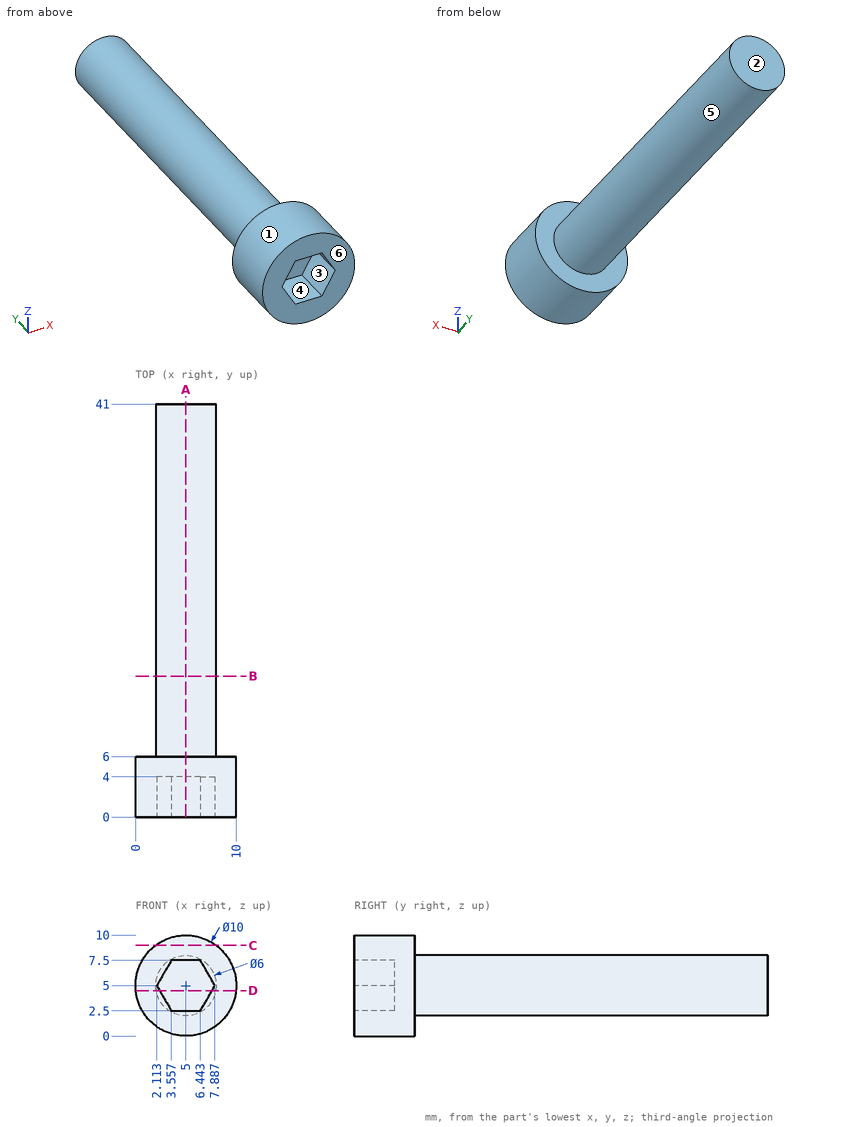
Geometry: see drawing. Coordinates: mm, zero at the bounding-box minimum. A direction names the side the tool comes from. Round coordinates to 2 decimals unless told otherwise and drop trailing zeros. Loops run counter-clockwise (first coordinate to the right, second up) from the corner with the lowest first, then second, coordinate; pieces in that order, holes last. Notation, with made-up numbers: (82, 79) - (130, 79) arc R27 cw to (130, 100) - close; hole circle Ø9 at (2.5, 38). An arc over 180 degrees is marked (long way). Write item = value, one per line. Start each with the question number.
(1) Set-up query: the marked faces 4, 5 and 6. Return all of +Z, -Z, +X, -X, +Y, -Y with unobstructed straight access to the full face (end or side cutting, diameter ignored); none if empty.
(2) Section query C-C, the plane z = 9. Output: boundary loops of the cut face in (x, y).
(3) Section query A-A, the plane x = 5. Output: boundary loops of the cut face in (y, z), plus the area to 3 significant figures.
(4) Section query B-B, the plane y = 14. Output: boundary loops of the cut face in (x, z).
(5) Pull-direction query (X, two-part tool) for the marked faces 1, 2 and 3; classes: +X half, -X half, draft (parallel to the pull), parting line (faces both ways), or undercut.
(6) Ray query, line 1 along Y through (x, z) = (7.25, 2.25); line 2 along Y through (x, z) = (3.75, 5.25); line 3 along X through (y, z) = (31, 5). Return the intervals inside material, ascending. Write a range as from..to.
(7) Pin query (flat end, axial travel): pin 1 (1 mm diameter, centred on x = 4.5, y = 16, fed in from -Z); pin 2 (1.5 mm diameter, centred on x = 4.5, z = 3.5, fed in from -Y); pin 3 (1 mm diameter, centred on x = 6, y = 11.5, fed in from +Z). Return the tip coordinate at first contact, or that it passes through.
(8) Section query D-D, the plane z = 4.5. Output: boundary loops of the cut face in (x, y) (1 decimal), plus the area to 3 significant figures.
Conclusion:
q1.face_4 = -Y
q1.face_5 = +Y
q1.face_6 = +Z, -Z, +X, -X, -Y
q2.outline = (2, 0) - (8, 0) - (8, 6) - (2, 6) - close
q3.outline = (0, 0) - (6, 0) - (6, 2) - (41, 2) - (41, 8) - (6, 8) - (6, 10) - (0, 10) - (0, 7.5) - (4, 7.5) - (4, 2.5) - (0, 2.5) - close
q3.area = 250 mm2
q4.outline = circle Ø6 at (5, 5)
q5.face_1 = parting line
q5.face_2 = draft
q5.face_3 = undercut
q6.line_1 = 0..6
q6.line_2 = 4..41
q6.line_3 = 2..8
q7.pin_1 = 2
q7.pin_2 = 4
q7.pin_3 = 7.96
q8.outline = (0, 0) - (2.4, 0) - (2.4, 4) - (7.6, 4) - (7.6, 0) - (10, 0) - (10, 6) - (8, 6) - (8, 41) - (2, 41) - (2, 6) - (0, 6) - close
q8.area = 246 mm2
